Build history of the part. All positions in model axes, mm. Give positions to 0.01 mm unless a question says otherwise; leave off trailing zeros. Order: outer loops, then holes, each group sorted by start corner. A loop starts at its lowest first (then second) coordinate and runs counter-clockwise, first axis right, second up. Notation, with made-up numbers: (-11.75, 71.25) -> (26.25, 71.25) arc R26 ccw to (26.25, 104.25) -> close; hole circle Ø4 at (-16.75, 38). An arc over 180 degrees is marked (long way). Use a Markdown table: item, result. Add a question column.
```python
from build123d import *

# Parameters (mm, degrees)
SKETCH1_W               = 300
SKETCH1_H               = 120
BOSS_EXTRUDE1_DEPTH     = 5
TAP_DRILL_FOR_M2_TAP1_D = 1.6
M3_CLEARANCE_HOLE1_D    = 3.2
SKETCH2_R               = 4.15
CUT_EXTRUDE1_DEPTH      = 324.148572641


with BuildPart() as part:
    # Sketch1 → Boss-Extrude1 (new body)
    with BuildSketch(Plane(origin=(0, 0, 0), x_dir=(1, 0, 0), z_dir=(0, 1, 0))):
        with Locations((150, -60)):
            Rectangle(SKETCH1_W, SKETCH1_H)
    extrude(amount=BOSS_EXTRUDE1_DEPTH)

    # Tap Drill for M2 Tap1 (through all)
    with Locations(Plane(origin=(0, 5, 0), x_dir=(1, 0, 0), z_dir=(0, 1, 0))):
        with Locations((113.641894276, -112.9946), (180.474494276, -112.9946), (180.474494276, -22.4976), (113.641894276, -22.4976)):
            Hole(TAP_DRILL_FOR_M2_TAP1_D / 2)

    # M3 Clearance Hole1 (through all)
    with Locations(Plane(origin=(0, 5, 0), x_dir=(1, 0, 0), z_dir=(0, 1, 0))):
        with Locations((92.641894276, -105), (92.641894276, -24), (189.641894276, -24), (189.641894276, -105)):
            Hole(M3_CLEARANCE_HOLE1_D / 2)

    # Sketch2 → Cut-Extrude1 (cut, through all)
    with BuildSketch(Plane(origin=(0, 5, 0), x_dir=(1, 0, 0), z_dir=(0, 1, 0))):
        with Locations(Location((15, -27, 0), (0, 0, 270))):
            Circle(SKETCH2_R)
        with Locations(Location((285, -27, 0), (0, 0, 90))):
            Circle(SKETCH2_R)
        with Locations(Location((285, -93, 0), (0, 0, 270))):
            Circle(SKETCH2_R)
        with Locations(Location((15, -93, 0), (0, 0, 90))):
            Circle(SKETCH2_R)
    extrude(amount=-CUT_EXTRUDE1_DEPTH, mode=Mode.SUBTRACT)


solid = part.part
```
(1) Mould opens along Z. For faces 1 (the face through (14.818, 2.535, 97.146)), 2 (the face through (148, 2, 120)), 3 (the face through (300, 2, 61)) say: released by +Z, released by -Z, zero draft, split by the parting line, or undercut.
(2) Band-saw the part on A-A on x = 285. Give the cut face in (y, z).
(3) Band-saw the part on B-B on z = 93. Give the cut face in (x, y), plus the area to 3 significant figures.
(4) Wall check: probe 1 along X at (y, z) = (3.7, 27); probe 2 along Z at (x, y) = (285, 3.85); probe 3 along Z at (x, y) = (93, 1.25). Give the ranges that are in metal, low to high.
(5) Pin check, flat tips, straight feed: pin 1 Ø9.5 at (x, z) = (15, 27) entering from +Y; pin 2 Ø7.5 at (x, z) = (285, 27) entering from -Y. Stop position of each tip, or through.
Response:
| question | item | result |
|---|---|---|
| 1 | face 1 | undercut |
| 1 | face 2 | released by +Z |
| 1 | face 3 | zero draft |
| 2 | outline | (0, 0) -> (5, 0) -> (5, 22.85) -> (0, 22.85) -> close; (0, 31.15) -> (5, 31.15) -> (5, 88.85) -> (0, 88.85) -> close; (0, 97.15) -> (5, 97.15) -> (5, 120) -> (0, 120) -> close |
| 3 | outline | (0, 0) -> (10.85, 0) -> (10.85, 5) -> (0, 5) -> close; (19.15, 0) -> (280.85, 0) -> (280.85, 5) -> (19.15, 5) -> close; (289.15, 0) -> (300, 0) -> (300, 5) -> (289.15, 5) -> close |
| 3 | area | 1,420 mm² |
| 4 | probe 1 | x = 0 to 10.85, 19.15 to 280.85, 289.15 to 300 |
| 4 | probe 2 | z = 0 to 22.85, 31.15 to 88.85, 97.15 to 120 |
| 4 | probe 3 | z = 0 to 22.44, 25.56 to 103.44, 106.56 to 120 |
| 5 | pin 1 | stops at y = 5 |
| 5 | pin 2 | passes through |
